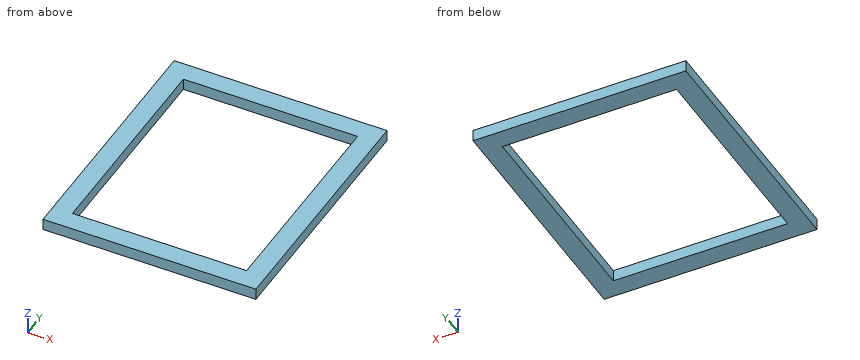
from build123d import *

# Parameters (mm, degrees)
F2_W = 50
F2_H = 30


with BuildPart() as f1:
    # F1: sweep along a path in F0
    with BuildLine(Plane.XY) as f1_path:
        Line((250, 300), (250, -300))
        Line((250, -300), (-250, -300))
        Line((-250, -300), (-250, 300))
        Line((-250, 300), (250, 300))
    # F2 (on Front) → F1 (sweep)
    with BuildSketch(Plane.XZ):
        with Locations((250, 0)):
            Rectangle(F2_W, F2_H)
    sweep(path=f1_path.line, transition=Transition.RIGHT)


solid = f1.part
Model file for the job. Use its own axes, mm. Give positions to 0.01 mm unless a question says otherwise; leave off trailing zeros. Write each loop counter-clockwise with the first axis right and the second up, starting at its lowest first coordinate (ties: lowest second). Pieces come first, ordered by that corner, then holes. Notation, with made-up numbers: (64.5, -33) -> (99.5, -33) arc R31 cw to (99.5, -4) -> close; hole circle Ø3 at (-30.5, 77.25). An arc over 180 degrees is marked (long way). Write item = value, one per line.
(1) Slice it at A-A, the plane x = -64.5. Give the cut face in (y, z), then the cut area to 3 significant figures.
Determined:
outline = (-325, -15) -> (-275, -15) -> (-275, 15) -> (-325, 15) -> close; (275, -15) -> (325, -15) -> (325, 15) -> (275, 15) -> close
area = 3,000 mm2
(2) Slice it at C-C, the plane z = 8. Give the cut face in (x, y).
Determined:
outline = (-275, -325) -> (275, -325) -> (275, 325) -> (-275, 325) -> close; hole (-225, -275) -> (225, -275) -> (225, 275) -> (-225, 275) -> close
(3) Probe line 1 along Y through (x, z) = (-32, 5); line 2 along X through (y, z) = (144.5, -10). List the from-to ranges inside material, lowest first.
Determined:
line_1 = -325 to -275, 275 to 325
line_2 = -275 to -225, 225 to 275
(4) Slice it at B-B, the plane y = 40.5. Give the cut face in (x, z).
Determined:
outline = (-275, -15) -> (-225, -15) -> (-225, 15) -> (-275, 15) -> close; (225, -15) -> (275, -15) -> (275, 15) -> (225, 15) -> close
